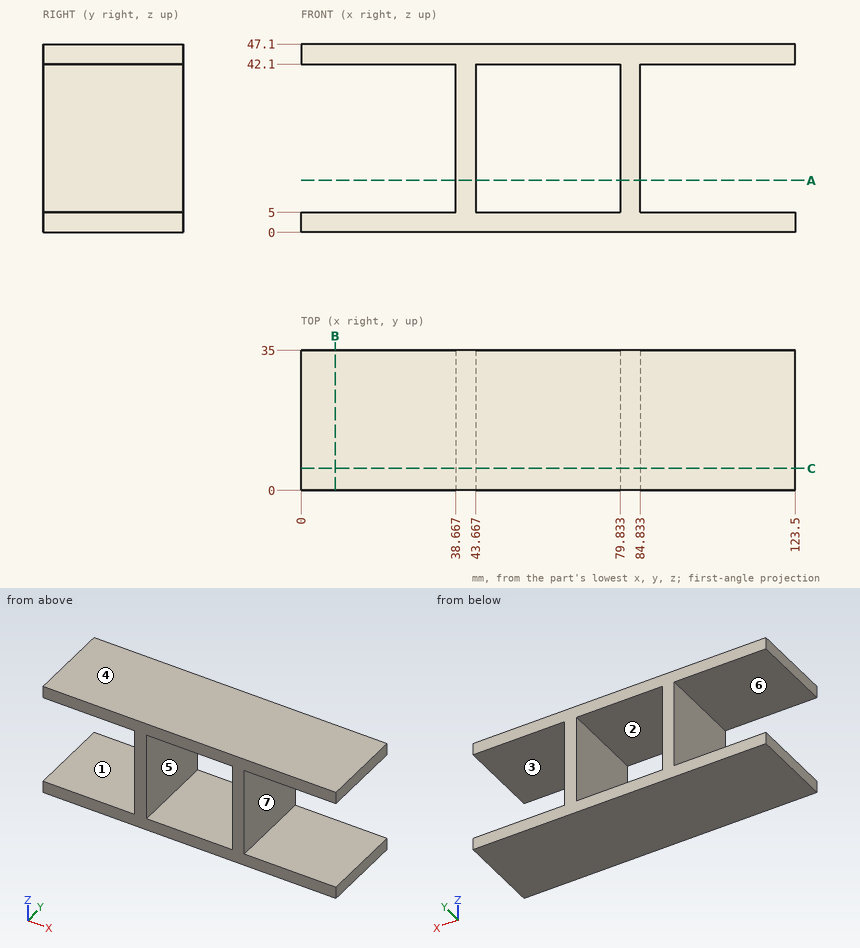
Geometry check sheet. Reference: drawing and pictorial views, mm from the part's lowest x, y, z. A direction names the side the tool comes from. Round coordinates to 2 decimals unless told otherwise and drop trailing zeros. Loops run counter-clockwise (first coordinate to the right, second up) from the corner with the lowest first, then second, coordinate; pieces in that order, holes last.
1. Scan lines: probe 1 along X at (y, z) = (5, 38); probe 2 along Z at (x, y) = (17.5, 7.5). Record each from-to range of solid material in increasing order.
2. Mould release check, pull along X, two halves, no side actions. Record for the marked faces 5, 6 and 7: released by +X, released by -X, zero draft, split by the parting line, or undercut.
3. Set-up check for the marked faces 1, 2, 3 and 4: record each of +Z, -Z, +X, -X, +Y, -Y from which the full face is reachable in a straight line by a thin tool's end or side.
4. Sectioned sample at B-B on x = 8.5. Record the boundary of the cut face in (y, z), and give its area (3 significant figures).
5. Sectioned sample at A-A on z = 13. Record the boundary of the cut face in (x, y), and give its area (3 significant figures).
6. Gauge pin test, flat ends, axial feed: pin 1 Ø4 at (x, y) = (35.5, 18) entering from -Z; pin 2 Ø8 at (y, z) = (8.5, 37) entering from +X. Record the tip position at first contact, or that the pin passes through.
7. Sectioned sample at C-C on y = 5.5. Record the boundary of the cut face in (x, z), and give its area (3 significant figures).
Recorded:
1. probe 1: x = 38.67 to 43.67, 79.83 to 84.83
1. probe 2: z = 0 to 5, 42.1 to 47.1
2. face 5: undercut
2. face 6: zero draft
2. face 7: released by +X
3. face 1: -X, +Y, -Y
3. face 2: +Y, -Y
3. face 3: +X, +Y, -Y
3. face 4: +Z, +X, -X, +Y, -Y
4. outline: (0, 0) - (35, 0) - (35, 5) - (0, 5) - close; (0, 42.1) - (35, 42.1) - (35, 47.1) - (0, 47.1) - close
4. area: 350 mm2
5. outline: (38.67, 0) - (43.67, 0) - (43.67, 35) - (38.67, 35) - close; (79.83, 0) - (84.83, 0) - (84.83, 35) - (79.83, 35) - close
5. area: 350 mm2
6. pin 1: stops at z = 0
6. pin 2: stops at x = 84.83
7. outline: (0, 0) - (123.5, 0) - (123.5, 5) - (84.83, 5) - (84.83, 42.1) - (123.5, 42.1) - (123.5, 47.1) - (0, 47.1) - (0, 42.1) - (38.67, 42.1) - (38.67, 5) - (0, 5) - close; hole (43.67, 5) - (79.83, 5) - (79.83, 42.1) - (43.67, 42.1) - close
7. area: 1,610 mm2
